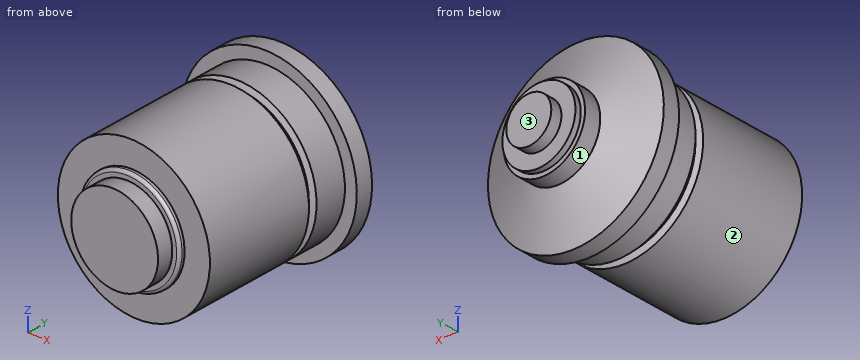
from build123d import *

# Parameters (mm, degrees)
FILLET1_R = 0.508


with BuildPart() as part:
    # Sketch1 → Revolve1 (revolve)
    with BuildSketch(Plane.XY, mode=Mode.PRIVATE) as revolve1_sk:
        Polygon((6.488, 39.7), (7.25, 39.7), (7.25, 36.7), (15.6125, 33.447007876), (15.6125, 30.440205684), (13.5, 30.440205684), (13.5, 3.8), (9, 3.8), (9, 2.8), (7.71, 2.8), (7.71, 0), (0, 0), (0, 42.748), (4, 42.748), (4, 40.748), (6.488, 40.748), align=None)
    revolve(revolve1_sk.sketch.rotate(Axis((0, 42.748, 0), (0, -1, 0)), 90), axis=Axis((0, 42.748, 0), (0, -1, 0)))

    # Sketch2 → Cut-Revolve1 (revolve, cut)
    with BuildSketch(Plane.XY, mode=Mode.PRIVATE) as cut_revolve1_sk:
        with BuildLine():
            Line((-13.5, 24.840205684), (-12.484, 24.471205684))
            Line((-12.484, 24.471205684), (-12.484, 23.709205684))
            Line((-12.484, 23.709205684), (-13.5, 23.340205684))
            ThreePointArc((-13.5, 23.340205684), (-14.429321734, 24.090205684), (-13.5, 24.840205684))
        make_face()
    revolve(cut_revolve1_sk.sketch.rotate(Axis((0, 0, 0), (0, 1, 0)), 270), axis=Axis((0, 0, 0), (0, 1, 0)), mode=Mode.SUBTRACT)

    # Fillet1
    fillet1_edges = [part.edges().sort_by_distance(p)[0] for p in [
        (0, 2.8, -9),
    ]]
    fillet(fillet1_edges, radius=FILLET1_R)


solid = part.part
Source: CAD feature listing. Evaluate the final solid. Frame: model axes, mm. Face numbers are marked on the shaded views. A direction names the side the tool comes from. Round coordinates to 2 decimals unless told otherwise and drop trailing zeros. Loops run counter-clockwise (first coordinate to the right, second up) from the corner with the lowest first, then second, coordinate; pieces in that order, holes last. Notation, with made-up numbers: M -35.5,71 L -23.5,71 A25 cw -23.5,99 Z; hole C 70.25,59 d7. An arc over 180 degrees is marked long. Answer as CSV lines item,"result".
Q1. Line query: line 1 along Y through (x, z) = (1, -4); line 2 along X through (y, z) = (6, -10.5); line 3 along Y through (x, z) = (13, -1.5). Output: solid intervals per line, ascending.
Verdict:
line 1,"y = 0 to 40.75"
line 2,"x = -8.49 to 8.49"
line 3,"y = 3.8 to 23.49, 24.69 to 34.43"
Q2. Cut plane A-A (y = 37.5). Return the cut outline in (x, z).
Verdict:
outline,"C 0,0 d14.5"
Q3. Contact query for flat-ended pins moving along their axis: pin 1 (4 mm diameter, centred on y = 23.5, z = 0, fed in from +X); pin 2 (12 mm diameter, centred on y = 9.5, z = -9, fed in from +X); pin 3 (12 mm diameter, centred on x = -7.5, y = 37, fed in from +Z). Output: stop coordinate, or through.
Verdict:
pin 1,"stops at x = 13.5"
pin 2,"stops at x = 13.16"
pin 3,"stops at z = 15.38"
Q4. Reachability of the marked faces 1, 2 and 3 from +Z, -Z, +X, -X, +Y, -Y: full face, straight path, thin tool, end or side. Return the list, or none.
Verdict:
face 1,"+Y"
face 2,"-Y"
face 3,"+Z, -Z, +X, -X, +Y"
Q5. Cut plane B-B (y = 17). Return the cut outline in (x, z), plus the area to 3 significant figures.
Verdict:
outline,"C 0,0 d27"
area,"573 mm^2"
